```python
from build123d import *

# Parameters (mm, degrees)
SKETCH1_W           = 30
SKETCH1_H           = 8.84
BOSS_EXTRUDE1_DEPTH = 12.75
DRAFT1_ANGLE        = 5


with BuildPart() as part:
    # Sketch1 → Boss-Extrude1 (new body)
    with BuildSketch(Plane(origin=(0, 0, 0), x_dir=(1, 0, 0), z_dir=(0, 1, 0))):
        with BuildLine():
            Line((14, -8.42), (-14, -8.42))
            ThreePointArc((-14, -8.42), (-17.535533906, -6.955533906), (-19, -3.42))
            Line((-19, -3.42), (-19, 3.42))
            ThreePointArc((-19, 3.42), (-17.535533906, 6.955533906), (-14, 8.42))
            Line((-14, 8.42), (14, 8.42))
            ThreePointArc((14, 8.42), (17.535533906, 6.955533906), (19, 3.42))
            Line((19, 3.42), (19, -3.42))
            ThreePointArc((19, -3.42), (17.535533906, -6.955533906), (14, -8.42))
        make_face()
        Rectangle(SKETCH1_W, SKETCH1_H, mode=Mode.SUBTRACT)
    extrude(amount=BOSS_EXTRUDE1_DEPTH)

    # Draft1
    draft1_faces = [part.faces().sort_by_distance(p)[0] for p in [
        (-17.535533906, 6.375, 6.955533906),
        (-19, 6.375, 0),
        (-17.535533906, 6.375, -6.955533906),
        (0, 6.375, -8.42),
        (17.535533906, 6.375, -6.955533906),
        (19, 6.375, 0),
        (17.535533906, 6.375, 6.955533906),
        (0, 6.375, 8.42),
    ]]
    draft(draft1_faces, Plane(origin=(-14, 12.75, 3.42), x_dir=(0, 0, 1), z_dir=(0, 1, 0)), DRAFT1_ANGLE)


solid = part.part
```
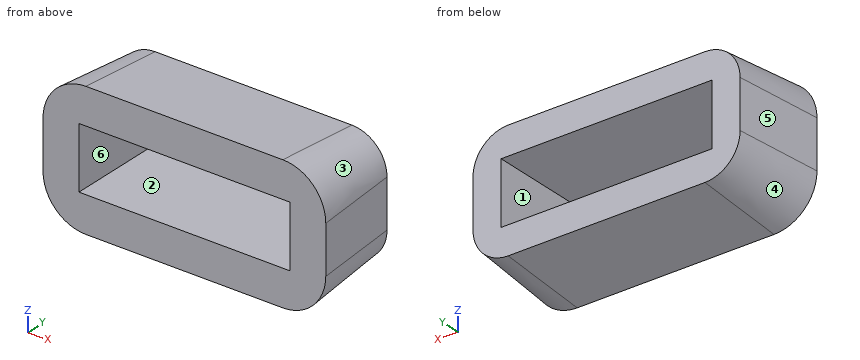
The listing builds one solid part. Answer for the finished solid, in the listing's coordinates (mm). Face numbers are marked on the shaded views. A direction names the side the tool comes from. Round coordinates to 2 decimals unless told otherwise and drop trailing zeros. Loops run counter-clockwise (first coordinate to the right, second up) from the corner with the lowest first, then second, coordinate; pieces in that order, holes last.
Q1. Section A-A, the plane x = 7 is taken. Determine the outline of the cut face in (y, z).
Q2. Section B-B, the plane z = -0.5 is taken. Determine the outline of the cut face in (x, y), then the cut area to 3 significant figures.
Q3. For a pull along X with two mould halves and no side action, classify the marked faces 1, 2, 3 and 4 as released by +X, released by -X, zero draft, split by the parting line, or undercut.
Q4. Section D-D, the plane y = 7 is taken. Determine the outline of the cut face in (x, z).
Q5. Find the intervals of material crossed by line 1 (Z direction, x = -8.5, y = 7.75); line 2 (X direction, y = 7, z = 2.5); line 3 (X direction, y = 9, z = -3.5), in increasing order.
Q6. Section C-C, the plane y = 3 is taken. Determine the outline of the cut face in (x, z).
Q7. Which of the six approach directions +Z, -Z, +X, -X, +Y, -Y give full straight-line access (tool end or side, diameter ignored) to the marked faces 5 and 6?
Q8. Given pin 1 Ø6 at (x, z) = (-3.5, 0.5) entering from -Y; pin 2 Ø4 at (x, y) = (3.5, 4) entering from -Z; pin 3 Ø7 at (y, z) = (8, 0) entering from -X; pin 4 Ø3 at (x, y) = (-2, 10.5) entering from +Z, each flat-ended and moving along its own axis, determine where each tip first touches the part or whether it passes through.
Completed:
1. outline: (0, -9.54) - (12.75, -8.42) - (12.75, -4.42) - (0, -4.42) - close; (0, 4.42) - (12.75, 4.42) - (12.75, 8.42) - (0, 9.54) - close
2. outline: (-20.12, 0) - (-15, 0) - (-15, 12.75) - (-19, 12.75) - close; (15, 0) - (20.12, 0) - (19, 12.75) - (15, 12.75) - close
2. area: 116 mm2
3. face 1: undercut
3. face 2: undercut
3. face 3: released by +X
3. face 4: released by -X
4. outline: (-19.5, -3.42) arc R5.5 ccw to (-14, -8.92) - (14, -8.92) arc R5.5 ccw to (19.5, -3.42) - (19.5, 3.42) arc R5.5 ccw to (14, 8.92) - (-14, 8.92) arc R5.5 ccw to (-19.5, 3.42) - close; hole (-15, -4.42) - (15, -4.42) - (15, 4.42) - (-15, 4.42) - close
5. line 1: z = -8.86 to -4.42, 4.42 to 8.86
5. line 2: x = -19.5 to -15, 15 to 19.5
5. line 3: x = -19.33 to -15, 15 to 19.33
6. outline: (-19.85, -3.42) arc R5.85 ccw to (-14, -9.27) - (14, -9.27) arc R5.85 ccw to (19.85, -3.42) - (19.85, 3.42) arc R5.85 ccw to (14, 9.27) - (-14, 9.27) arc R5.85 ccw to (-19.85, 3.42) - close; hole (-15, -4.42) - (15, -4.42) - (15, 4.42) - (-15, 4.42) - close
7. face 5: +Z, -Z, -X, +Y
7. face 6: +Y, -Y
8. pin 1: passes through
8. pin 2: stops at z = -9.36
8. pin 3: stops at x = -19.72
8. pin 4: stops at z = 8.75
